```python
from build123d import *

# Parameters (mm, degrees)
F0_W        = 17.0710533857
F0_H        = 167.5858162344
F1_DEPTH    = 7.62
F2_W        = 17.0710533857
F2_H        = 17.0666188933
F3_DEPTH    = 5.08
F4_T1_DEPTH = 92.8391963602


# Not quite as in the source:
# - a fillet or chamfer that OpenCascade refuses, or shapes differently, is made with other operations: its cross-section is extruded or revolved along the edge and cut away or added


with BuildPart() as f1:
    # F0 (on Top) → F1 (new body)
    with BuildSketch(Plane.XY):
        with Locations((-152.5016650558, 70.9913838655)):
            Rectangle(F0_W, F0_H)
        Polygon((-168.1138426065, 171.4205145836), (-161.0371917486, 154.7842919827), (-143.9661383629, 154.7842919827), (-136.3786160946, 170.9794849157), (-136.3786160946, 192.3550665379), (-171.417593956, 192.3550665379), align=None)
    extrude(amount=F1_DEPTH)

    # F2 (on face) → F3 (join)
    with BuildSketch(Plane(origin=(0, 0, 0), x_dir=(1, 0, 0), z_dir=(0, 0, -1))):
        with Locations((-152.5016650558, 4.2682148051)):
            Rectangle(F2_W, F2_H)
    extrude(amount=F3_DEPTH)

    # F4: fillet of radius 25.1416200386 on 1 edges, made by hand

    # F4_s2 → F4_t1 (cut)
    with BuildSketch(Plane.YZ.offset(-198.9212632358)):
        with BuildLine():
            ThreePointArc((4.2650946416, 0), (-2.8973065821, -3.7761932686), (-10.8885339533, -5.08))
            Line((-10.8885339533, -5.08), (-10.8885339533, -5.5828324008))
            Line((-10.8885339533, -5.5828324008), (4.2650946416, -5.5828324008))
            Line((4.2650946416, -5.5828324008), (4.7679270424, -5.08))
            ThreePointArc((4.7679270424, -5.08), (4.7679270424, -2.54), (4.5681672135, -0.4012324008))
            Line((4.5681672135, -0.4012324008), (4.2650946416, 0))
        make_face()
    extrude(amount=F4_T1_DEPTH, mode=Mode.SUBTRACT)


solid = f1.part
```
Can you work these out from the model? Positions are in its coordinate system, mm. A direction names the side the tool comes from. Coordinates: 2 decimals unless noted, no trailing zeros. Loops run counter-clockwise (first coordinate to the right, second up) from the corner with the lowest first, then second, coordinate; pieces in that order, holes last. Notation, with made-up numbers: M -5.5,13.5 L -1.5,13.5 A20 ccw -1.5,26.5 Z; hole C -20.5,-32 d3. An arc over 180 degrees is marked long. Put each result on its own line as item: value. Start each with the question number.
(1) Which directions (+Z, -Z, +X, -X, +Y, -Y) give clear straight access to the entire face, cutting with the end or side of a thin tool? Please do faces 1 (the face through (-161.037, 72, 4)), 2 (the face through (-154, 121, 0)), 3 (the face through (-143.966, 72, 4)).
(2) Will these pins go through, and if not, where does the flat tip stop? pin 1 Ø4 at (x, y) = (-144.5, 51.5) entering from -Z; pin 2 Ø6.5 at (y, z) = (66.5, -0.5) entering from +X; pin 3 Ø6 at (y, z) = (130, 0.5) entering from -X.
(3) Imagine slicing it at B-B on x = -149. List the corners of the cut face in (y, z) for me, and give its area (3 significant figures).
(4) Imagine slicing it at C-C on y = 141. List the corners of the cut face in (x, z) for me.
(5) I need wall thicknesses on probe 1 along X at (y, z) = (54, 5.75); probe 2 along Z at (x, y) = (-160, 90); probe 3 along X at (y, z) = (158, 6). Which ranges of each line are inside material? Lowest first, please.
(6) Imagine slicing it at D-D on z = -3.25. List the corners of the cut face in (x, y) for me.
(7) Imagine slicing it at A-A on z = 5. List the corners of the cut face in (x, y) for me, and give its area (3 significant figures).
Worked answers:
1. face 1: +Z, -Z, -X, -Y
1. face 2: -Z, +X, -X, +Y
1. face 3: +Z, -Z, +X, -Y
2. pin 1: stops at z = 0
2. pin 2: stops at x = -143.97
2. pin 3: stops at x = -161.04
3. outline: M -12.8,-5.08 L -10.89,-5.08 A25.14 ccw 4.27,0 L 192.36,0 L 192.36,7.62 L -12.8,7.62 Z
3. area: 1,630 mm2
4. outline: M -161.04,0 L -143.97,0 L -143.97,7.62 L -161.04,7.62 Z
5. probe 1: x = -161.04 to -143.97
5. probe 2: z = 0 to 7.62
5. probe 3: x = -162.41 to -142.46
6. outline: M -161.04,-12.8 L -143.97,-12.8 L -143.97,-1.47 L -161.04,-1.47 Z
7. outline: M -171.42,192.36 L -168.11,171.42 L -161.04,154.78 L -161.04,-12.8 L -143.97,-12.8 L -143.97,154.78 L -136.38,170.98 L -136.38,192.36 Z
7. area: 3,970 mm2
